Build history of the part. All positions in model axes, mm. A direction names the side the tool comes from. Round coordinates to 2 decimals unless told otherwise and drop trailing zeros. Write each loop counter-clockwise with the first axis right and the second up, starting at its lowest first coordinate (ties: lowest second). Pieces come first, ordered by that corner, then holes.
Item 1: Band-saw the part on B-B, the plane z = 13.25. Write the cut outline in (x, y) (3 decimals).
Item 2: Wall check: probe 1 along Y at (x, z) = (-7.5, 0.45) (3 decimals); probe 2 along X at (y, z) = (1.75, 5.25); probe 3 along X at (y, z) = (-0.5, 2.25). Give the ranges that are in metal, low to high.
Item 3: Drop flat-ended pins along their axis: pin 1 Ø1 at (x, y) = (5, -4.5) entering from +Z (3 decimals); pin 2 Ø9.5 at (x, y) = (22.225, -3.175) entering from -Z. Give the stop position or say it passes through.
Item 4: Band-saw the part on A-A, the plane x = 7.5. Write the cut outline in (y, z) (3 decimals), then the cut area to 3 significant figures.
Item 5: Mould opens along Y. For faces 1 (the cylindrical face through (3.746, 0.165, 0.939)), 2 (the cylindrical face through (27.46, 8.8, 9.78)), 3 (the flat face through (28.224, 0, 10)) say: +Y half, -Y half, draft (parallel to the pull), parting line (faces both ways), or undercut.
Item 6: 3-axis set-ups, long thin cutter, end or side, ignore diameter. For faces 4 (the flat face through (22, 0, 19.05)), 5 (the cylindrical face through (16.99, -8.8, 10.36)), 6 (the flat face through (-16.226, 0, 11)), 7 (the cylindrical face through (-16.99, 8.8, 10.36)): which of +Z, -Z, +X, -X, +Y, -Y reach the whole face in a straight line?
Item 7: Band-saw the part on C-C, the plane x = 0. Write the cut outline in (y, z) (3 decimals), then the cut area to 3 significant figures.
```python
from build123d import *

# Parameters (mm, degrees)
SKETCH1_W           = 56.44896
SKETCH1_H           = 19.05
SKETCH1_R           = 2.99974
BOSS_EXTRUDE1_DEPTH = 19.05
SKETCH2_R           = 1.45
SKETCH2_R_2         = 3.75
CUT_EXTRUDE1_DEPTH  = 19.05
SKETCH3_W           = 32.45104
SKETCH3_H           = 17.145
CUT_EXTRUDE2_DEPTH  = 19.05
FILLET1_R           = 2.54
FILLET3_R           = 0.254


with BuildPart() as part:
    # Sketch1 → Boss-Extrude1 (new body)
    with BuildSketch(Plane.XY):
        Rectangle(SKETCH1_W, SKETCH1_H)
        with Locations((-22.225, -3.175)):
            Circle(SKETCH1_R, mode=Mode.SUBTRACT)
        with Locations((22.225, -3.175)):
            Circle(SKETCH1_R, mode=Mode.SUBTRACT)
    extrude(amount=BOSS_EXTRUDE1_DEPTH)

    # Sketch2 → Cut-Extrude1 (cut)
    with BuildSketch(Plane(origin=(0, 0, 0), x_dir=(-1, 0, 0), z_dir=(0, 0, -1))):
        with Locations((-7.5, 0)):
            Circle(SKETCH2_R)
        with Locations((7.5, 0)):
            Circle(SKETCH2_R)
        Circle(SKETCH2_R_2)
    extrude(amount=-CUT_EXTRUDE1_DEPTH, mode=Mode.SUBTRACT)

    # Sketch3 → Cut-Extrude2 (cut)
    with BuildSketch(Plane(origin=(0, 9.525, 0), x_dir=(1, 0, 0), z_dir=(0, 1, 0))):
        with Locations((0, -10.4775)):
            Rectangle(SKETCH3_W, SKETCH3_H)
    extrude(amount=-CUT_EXTRUDE2_DEPTH, mode=Mode.SUBTRACT)

    # Fillet1
    fillet1_edges = [part.edges().sort_by_distance(p)[0] for p in [
        (28.22448, -9.525, 9.525),
        (-28.22448, -9.525, 9.525),
        (-28.22448, 9.525, 9.525),
        (28.22448, 9.525, 9.525),
        (16.22552, -9.525, 10.4775),
        (16.22552, 9.525, 10.4775),
        (-16.22552, 9.525, 10.4775),
        (-16.22552, -9.525, 10.4775),
    ]]
    fillet(fillet1_edges, radius=FILLET1_R)

    # Fillet3
    fillet3_edges = [part.edges().sort_by_distance(p)[0] for p in [
        (0, -9.525, 0),
        (28.22448, 0, 0),
        (-28.22448, 0, 0),
        (0, 9.525, 0),
        (-27.480531224, 8.781051224, 0),
        (27.480531224, 8.781051224, 0),
        (27.480531224, -8.781051224, 0),
        (-27.480531224, -8.781051224, 0),
    ]]
    fillet(fillet3_edges, radius=FILLET3_R)


solid = part.part
```
Results:
1. outline: (-28.224, -6.985) arc R2.54 ccw to (-25.684, -9.525) - (-18.766, -9.525) arc R2.54 ccw to (-16.226, -6.985) - (-16.226, 6.985) arc R2.54 ccw to (-18.766, 9.525) - (-25.684, 9.525) arc R2.54 ccw to (-28.224, 6.985) - close; (16.226, -6.985) arc R2.54 ccw to (18.766, -9.525) - (25.684, -9.525) arc R2.54 ccw to (28.224, -6.985) - (28.224, 6.985) arc R2.54 ccw to (25.684, 9.525) - (18.766, 9.525) arc R2.54 ccw to (16.226, 6.985) - close; hole circle Ø5.999 at (-22.225, -3.175); hole circle Ø5.999 at (22.225, -3.175)
2. probe 1: y = -9.525 to -1.45, 1.45 to 9.525
2. probe 2: x = -28.22 to -16.23, 16.23 to 28.22
2. probe 3: x = -28.22 to -23.58, -20.87 to -16.23, 16.23 to 20.87, 23.58 to 28.22
3. pin 1: stops at z = 1.905
3. pin 2: stops at z = 0
4. outline: (-9.525, 0.254) arc R0.254 ccw to (-9.271, 0) - (-1.45, 0) - (-1.45, 1.905) - (-9.525, 1.905) - close; (1.45, 0) - (9.271, 0) arc R0.254 ccw to (9.525, 0.254) - (9.525, 1.905) - (1.45, 1.905) - close
4. area: 30.7 mm2
5. face 1: undercut
5. face 2: +Y half
5. face 3: draft
6. face 4: +Z, +X, -X, +Y, -Y
6. face 5: +Z, -Y
6. face 6: +Z, +Y, -Y
6. face 7: +Z, +Y
7. outline: (-9.525, 0.254) arc R0.254 ccw to (-9.271, 0) - (-3.75, 0) - (-3.75, 1.905) - (-9.525, 1.905) - close; (3.75, 0) - (9.271, 0) arc R0.254 ccw to (9.525, 0.254) - (9.525, 1.905) - (3.75, 1.905) - close
7. area: 22.0 mm2
